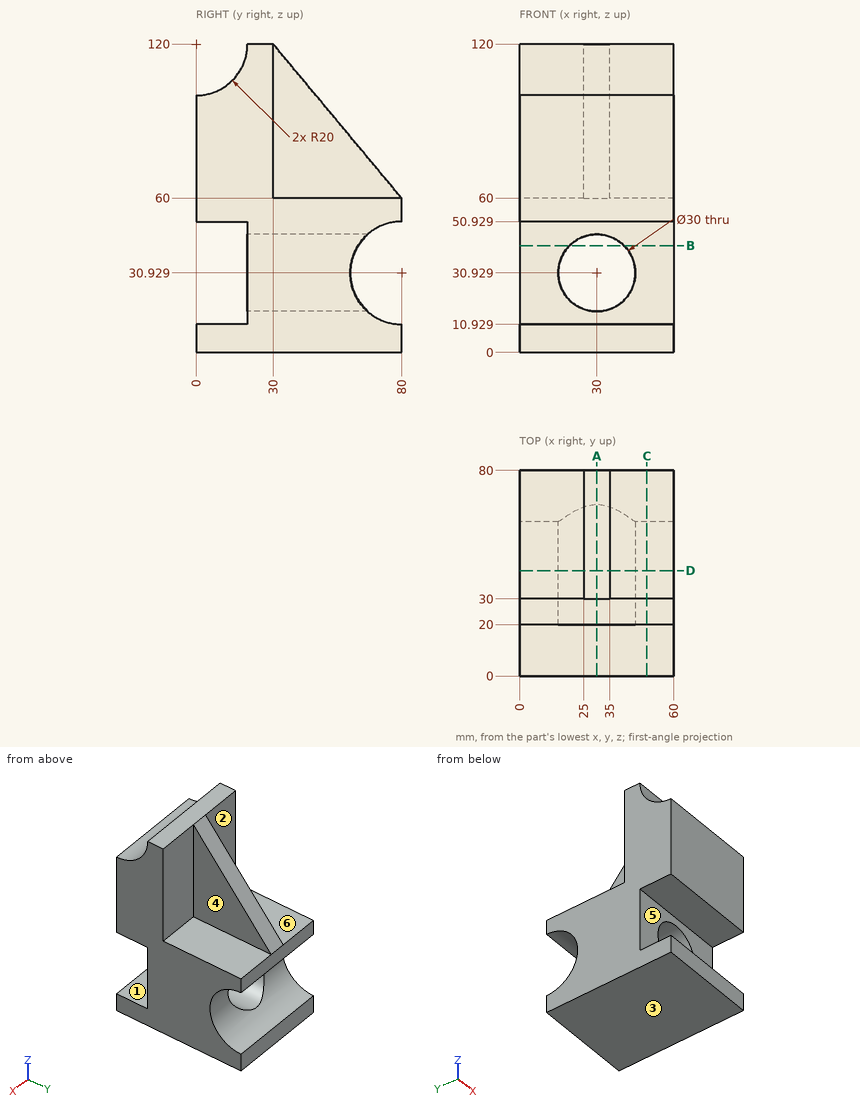
Design review of the part shown in the three views and the two pictorial views. Dimensions are in mm from the part's minimum x, y and z. A direction names the side the tool comes from. Coordinates: 2 decimals unless noted, no trailing zeros. Order: outer loops, then holes, each group sorted by start corner. A loop starts at its lowest first (then second) coordinate and runs counter-clockwise, first axis right, second up. Notation, with made-up numbers: (-9.5, 70.5) - (20.5, 70.5) arc R32 ccw to (20.5, 100.5) - close; hole circle Ø1 at (-22.75, 34.5). An arc over 180 degrees is marked (long way). Answer as CSV lines item,"result". Start each with the question number.
1) To check wall thickness, follow line 1 along Z through (x, y) = (49, 31.5); line 2 along Y through (x, z) = (58, 32); line 3 along X through (y, z) = (57.5, 19). State the ranges of each line that lie inside material, in increasing order. Write a range as [from, to].
2) Add section C-C (x = 49.5). State the section outline as (y, z) points, then the cut area to 3 significant figures.
3) Machinability: for the marked faces 4, 5 and 6, which of the approach directions +Z, -Z, +X, -X, +Y, -Y give a long, thin tool a straight path to every point of the face, cutting with its end or side? Answer none if there is none.
4) Add section B-B (z = 41.5). State the section outline as (x, y) points, then the cut area to 3 significant figures.
5) Draft analysis for pull direction Z (two halves, no side actions). For the marked faces 1, 2 and 3, state which applies: +Z half, -Z half, draft (parallel to the pull), parting line (faces both ways), or undercut.
6) Add section D-D (y = 41). State the section outline as (x, z) points, then the cut area to 3 significant figures.
7) Add section A-A (x = 30). State the section outline as (y, z) points, then the cut area to 3 significant figures.
8) Insertion check: P1, Ø1.5, axis at y = 65, z = 71, coming from the +X side; P2, Ø20, axis at x = 30, z = 39.5, coming from the -Y side; P3, Ø15, axis at y = 55, z = 93, coming from the -X side. Each pin has a flat end and moves straight along its axis. Give the tip position at first contact, or say it passes through.
Result:
1,line 1,"[0, 60]"
1,line 2,"[20, 60.03]"
1,line 3,"[0, 20.91], [39.09, 60]"
2,outline,"(0, 0) - (80, 0) - (80, 10.93) arc R20 cw to (80, 50.93) - (80, 60) - (30, 60) - (30, 120) - (20, 120) arc R20 cw to (0, 100) - (0, 50.93) - (20, 50.93) - (20, 10.93) - (0, 10.93) - close"
2,area,"4,860 mm^2"
3,face 4,"+Z, +X, +Y"
3,face 5,"+X, -X, -Y"
3,face 6,"+Z, -X, +Y"
4,outline,"(0, 20) - (19.36, 20) - (19.36, 63.02) - (0, 63.02) - close; (40.64, 20) - (60, 20) - (60, 63.02) - (40.64, 63.02) - close"
4,area,"1,670 mm^2"
5,face 1,"undercut"
5,face 2,"draft"
5,face 3,"-Z half"
6,outline,"(0, 0) - (60, 0) - (60, 60) - (35, 60) - (35, 106.8) - (25, 106.8) - (25, 60) - (0, 60) - close; hole circle Ø30 at (30, 30.93)"
6,area,"3,360 mm^2"
7,outline,"(0, 0) - (80, 0) - (80, 10.93) arc R20 cw to (66.77, 15.93) - (20, 15.93) - (20, 10.93) - (0, 10.93) - close; (0, 50.93) - (20, 50.93) - (20, 45.93) - (66.77, 45.93) arc R20 cw to (80, 50.93) - (80, 60) - (30, 120) - (20, 120) arc R20 cw to (0, 100) - close"
7,area,"5,100 mm^2"
8,P1,"x = 35"
8,P2,"y = 20"
8,P3,"x = 25"
